from build123d import *

# Parameters (mm, degrees)
F0_R     = 36.5
F0_R_2   = 2.794
F1_DEPTH = 3.81
F2_SIZE  = 1.27
F4_DEPTH = 17.78
F5_R     = 1.90499


# Not quite as in the source:
# - a fillet or chamfer is up to 0.001 mm smaller than in the source, because OpenCascade refuses the exact size


with BuildPart() as f1:
    # F0 (on Top) → F1 (new body)
    with BuildSketch(Plane.XY):
        Circle(F0_R)
        with Locations((-28.194, 0)):
            Circle(F0_R_2, mode=Mode.SUBTRACT)
        with Locations((28.194, 0)):
            Circle(F0_R_2, mode=Mode.SUBTRACT)
        with Locations((0, 28.194)):
            Circle(F0_R_2, mode=Mode.SUBTRACT)
    extrude(amount=F1_DEPTH)

    # F2
    f2_edges = [f1.edges().sort_by_distance(p)[0] for p in [
        (-36.5, 0, 0),
    ]]
    chamfer(f2_edges, length=F2_SIZE)

    # F3 (on face) → F4 (join)
    with BuildSketch(Plane(origin=(0, 0, 0), x_dir=(1, 0, 0), z_dir=(0, 0, -1))):
        with BuildLine():
            Line((16.51, 17.78), (16.51, 0))
            ThreePointArc((16.51, 0), (0, -16.51), (-16.51, 0))
            Line((-16.51, 0), (-16.51, 17.78))
            ThreePointArc((-16.51, 17.78), (-18.415, 19.685), (-20.32, 17.78))
            Line((-20.32, 17.78), (-20.32, 0))
            ThreePointArc((-20.32, 0), (0, -20.32), (20.32, 0))
            Line((20.32, 0), (20.32, 17.78))
            ThreePointArc((20.32, 17.78), (18.415, 19.685), (16.51, 17.78))
        make_face()
    extrude(amount=F4_DEPTH)

    # F5 (radius 1.905 in the source; OpenCascade refuses exactly that, so slightly less here)
    f5_edges = [f1.edges().sort_by_distance(p)[0] for p in [
        (-20.32, -8.89, -17.78),
        (-16.51, -8.89, -17.78),
        (-18.415, -19.685, -17.78),
        (0, 20.32, -17.78),
        (0, 16.51, -17.78),
        (16.51, -8.89, -17.78),
        (20.32, -8.89, -17.78),
        (18.415, -19.685, -17.78),
    ]]
    fillet(f5_edges, radius=F5_R)


solid = f1.part
Verification items for the finished model (mm, model axes). A direction names the side the tool comes from. Coordinates: 2 decimals unless noted, no trailing zeros. Write each loop counter-clockwise with the first axis right and the second up, starting at its lowest first coordinate (ties: lowest second). Pieces come first, ordered by that corner, then holes. Notation, with made-up numbers: (70, -26.5) - (80, -26.5) arc R22 ccw to (80, -19.5) - close; hole circle Ø5 at (-17, 69.25). An arc over 180 degrees is marked (long way). Answer as a JSON object with one key per item and string values.
(1) Thickness scan on line 1 along X through (y, z) = (-0.5, 3); line 2 along Z through (x, y) = (-14.5, 18.5); line 3 along X through (y, z) = (3.5, -16.25). Record the ranges inside material, lowest first.
Report:
{"line 1": "-36.5 to -30.94, -25.45 to 25.45, 30.94 to 36.5", "line 2": "0 to 3.81", "line 3": "-19.98 to -16.17, 16.17 to 19.98"}
(2) Gauge pin test, flat ends, axial feed: pin 1 Ø1 at (y, z) = (15.5, 0.5) entering from +X; pin 2 Ø2 at (x, y) = (19.5, 17) entering from -Z; pin 3 Ø12.5 at (y, z) = (-6, -11) entering from +X; pin 4 Ø3.5 at (x, y) = (-28.194, 0) entering from -Z. Record the tip position at first contact, or that the pin passes through.
Report:
{"pin 1": "x = 32.79", "pin 2": "z = 0", "pin 3": "x = 20.32", "pin 4": "through"}
(3) Cross-section at A-A on z = -11.75. Record the cut outline in (x, y) (3 decimals), plus the area to 3 significant figures.
Report:
{"outline": "(-20.32, -17.78) arc R1.905 ccw to (-16.51, -17.78) - (-16.51, 0) arc R16.51 cw to (16.51, 0) - (16.51, -17.78) arc R1.905 ccw to (20.32, -17.78) - (20.32, 0) arc R20.32 ccw to (-20.32, 0) - close", "area": "367 mm^2"}
(4) Tool access check on faces 4 (the flat face through (0, 0, 0)), 5 (the cylindrical face through (-17.053, -9.014, -17.207)), 6 (the flat face through (20.32, -9, -8)), 7 (the cylindrical face through (-0.447, 20.315, -7.826)). Record the directions out of +Z, -Z, +X, -X, +Y, -Y that give a thin tool (end or side, any length) a straight path to the whole face; none if there is none.
Report:
{"face 4": "-Z", "face 5": "-Z, -Y", "face 6": "-Z, +X, +Y, -Y", "face 7": "-Z, +Y"}
(5) Mould release check, pull along Z, two halves, no side actions. Record for faces 1 (the cylindrical face through (19.777, -9.014, -17.207)), 2 (the flat face through (-1, 1, 3.81)), 3 (the cylindrical face through (-30.985, 0.123, 1.878)): pulls with the +Z half, pulls with the -Z half, needs draft (parallel to the pull), parting line crosses it, or undercut.
Report:
{"face 1": "pulls with the -Z half", "face 2": "pulls with the +Z half", "face 3": "needs draft"}
